Read the model definition and answer for the solid it produces. Units are mm, in the model's axes. A direction names the side the tool comes from. Give positions to 0.01 mm unless a question says otherwise; leave off trailing zeros. Order: outer loops, then holes, each group sorted by start corner. A loop starts at its lowest first (then second) coordinate and runs counter-clockwise, first axis right, second up. Notation, with made-up numbers: (83, -7) - (114, -7) arc R22 ccw to (114, 14) - close; hole circle Ø10 at (47, -6.75). An arc over 180 degrees is marked (long way). Return JSON: item names as keys, results as strings.
```python
from build123d import *

# Parameters (mm, degrees)
F0_R           = 20.05
F1_DEPTH       = 3.1
F2_R           = 10.05
F3_DEPTH       = 2
F4_R           = 0.5
F6_R           = 6
F7_DEPTH       = 10
F8_R           = 4.05
F9_DEPTH       = 8
F10_DEPTH      = 10.001
F10_DEPTH_BACK = 3.1010001
F11_T1_DEPTH   = 15.3170452501
F11_T4_ANGLE   = 359.9586190749


# Not quite as in the source:
# - a fillet or chamfer that OpenCascade refuses, or shapes differently, is made with other operations: its cross-section is extruded or revolved along the edge and cut away or added


with BuildPart() as f1:
    # F0 (on Top) → F1 (new body)
    with BuildSketch(Plane.XY):
        Circle(F0_R)
    extrude(amount=F1_DEPTH)

    # F2 (on face) → F3 (cut)
    with BuildSketch(Plane.XY.offset(3.1)):
        Circle(F2_R)
    extrude(amount=-F3_DEPTH, mode=Mode.SUBTRACT)

    # F4
    f4_edges = [f1.edges().sort_by_distance(p)[0] for p in [
        (-20.05, 0, 3.1),
        (-10.05, 0, 3.1),
        (-20.05, 0, 0),
    ]]
    fillet(f4_edges, radius=F4_R)

    # F6 (on face) → F7 (join)
    with BuildSketch(Plane(origin=(0, 0, 0), x_dir=(1, 0, 0), z_dir=(0, 0, -1))):
        Circle(F6_R)
    extrude(amount=F7_DEPTH)

    # F8 (on face) → F9 (cut)
    with BuildSketch(Plane(origin=(0, 0, -10), x_dir=(1, 0, 0), z_dir=(0, 0, -1))):
        Circle(F8_R)
    extrude(amount=-F9_DEPTH, mode=Mode.SUBTRACT)

    # F5 (on face) → F10 (cut, two sides)
    with BuildSketch(Plane(origin=(0, 0, 0), x_dir=(1, 0, 0), z_dir=(0, 0, -1))) as f10_sk:
        with BuildLine():
            Line((-2.5, 5), (-2.5, 0))
            ThreePointArc((-2.5, 0), (0, -2.5), (2.5, 0))
            Line((2.5, 0), (2.5, 5))
            ThreePointArc((2.5, 5), (1.9142135624, 6.4142135624), (0.5, 7))
            Line((0.5, 7), (-0.5, 7))
            ThreePointArc((-0.5, 7), (-1.9142135624, 6.4142135624), (-2.5, 5))
        make_face()
    extrude(amount=F10_DEPTH, mode=Mode.SUBTRACT)
    extrude(f10_sk.sketch, amount=-F10_DEPTH_BACK, mode=Mode.SUBTRACT)

    # F11: fillet of radius 1 on 3 edges, made by hand

    # F11_s2 → F11_t1 (cut)
    with BuildSketch(Plane.XY.offset(-15.3170452501)):
        with BuildLine():
            ThreePointArc((-4.2, -4.2848570571), (-3.1127016654, -4.49266866), (-2.5, -3.5707142143))
            Line((-2.5, -3.5707142143), (-2.4, -3.5707142143))
            ThreePointArc((-2.4, -3.5707142143), (-2.4, -5), (-2.3442646941, -5.4568235306))
            Line((-2.3442646941, -5.4568235306), (-2.4820201112, -5.5722146555))
            ThreePointArc((-2.4820201112, -5.5722146555), (-3.4303168121, -5.0440981918), (-4.27, -4.3562713414))
            Line((-4.27, -4.3562713414), (-4.2, -4.2848570571))
        make_face()
        with BuildLine():
            ThreePointArc((4.2, -4.2848570571), (3.1127016654, -4.49266866), (2.5, -3.5707142143))
            Line((2.5, -3.5707142143), (2.4, -3.5707142143))
            ThreePointArc((2.4, -3.5707142143), (2.4, -5), (2.3442646941, -5.4568235306))
            Line((2.3442646941, -5.4568235306), (2.4820201112, -5.5722146555))
            ThreePointArc((2.4820201112, -5.5722146555), (3.4303168121, -5.0440981918), (4.27, -4.3562713414))
            Line((4.27, -4.3562713414), (4.2, -4.2848570571))
        make_face()
    extrude(amount=F11_T1_DEPTH, mode=Mode.SUBTRACT)

    # F11_s3 → F11_t4 (revolve, cut)
    with BuildSketch(Plane(origin=(0, 0, 0), x_dir=(0, 0, 1), z_dir=(-0.9999999348, -0.0003611167, 0))):
        with BuildLine():
            ThreePointArc((-10, -5), (-9.7071067812, -5.7071067812), (-9, -6))
            Line((-9, -6), (-10, -6))
            Line((-10, -6), (-10, -5))
        make_face()
    revolve(axis=Axis((0, 0, -10), (0, 0, 1)), revolution_arc=F11_T4_ANGLE, mode=Mode.SUBTRACT)


solid = f1.part
```
Q1. Given pin 1 (1.5 mm diameter, centred on y = -3, z = -2, fed in from +X); pin 2 (16 mm diameter, centred on x = 0, y = 0, fed in from +Z); pin 3 (1.5 mm diameter, centred on y = -3, z = -2, fed in from -X), each flat-ended and moving along its own axis, determine where each tip first touches the part or whether it passes through.
Values:
{"pin 1": "stops at x = 5.56", "pin 2": "stops at z = 1.1", "pin 3": "stops at x = -5.56"}
Q2. A cutting plane is placed at A-A (x = 0). Write down the section's boundary in (y, z), and give its area (3 significant figures).
Values:
{"outline": "(-20.05, 0.5) arc R0.5 ccw to (-19.55, 0) - (-7, 0) - (-7, 1.1) - (-10.05, 1.1) - (-10.05, 2.6) arc R0.5 ccw to (-10.55, 3.1) - (-19.55, 3.1) arc R0.5 ccw to (-20.05, 2.6) - close; (2.5, -2) - (4.05, -2) - (4.05, -10) - (5, -10) arc R1 ccw to (6, -9) - (6, 0) - (19.55, 0) arc R0.5 ccw to (20.05, 0.5) - (20.05, 2.6) arc R0.5 ccw to (19.55, 3.1) - (10.55, 3.1) arc R0.5 ccw to (10.05, 2.6) - (10.05, 1.1) - (2.5, 1.1) - close", "area": "95.7 mm²"}
Q3. For faces 5 (the flat face through (2.5, -2.3, -1.6)), 6 (the cylindrical face through (0, 6, -4)), 7 (the flat face through (8, -8, 3.1)), 8 (the cylindrical face through (-3.13, -4.5, -5.07)), 9 (the flat face through (2, 2, 1.1)), determine the directions among +Z, -Z, +X, -X, +Y, -Y from which every point of the face is accessible in a straight line to the end or side of a thin tool.
Values:
{"face 5": "+Z, -Z", "face 6": "-Z", "face 7": "+Z, +X, -X, +Y, -Y", "face 8": "-Z, -Y", "face 9": "+Z"}
Q4. A cutting plane is placed at B-B (z = -1). Write down the section's boundary in (x, y), and give its area (3 significant figures).
Values:
{"outline": "(-4.2, -4.28) arc R1 ccw to (-2.5, -3.57) - (-2.5, 0) arc R2.5 cw to (2.5, 0) - (2.5, -3.57) arc R1 ccw to (4.2, -4.28) arc R6 ccw (long way) to start", "area": "72.4 mm²"}
Q5. Consider L1, parallel to X at y = 0, z = -6; L2, parallel to Y at x = 0, z = 1.85; L3, parallel to Z at x = -7, y = 15. Determine where each line is inside the solid, lowest interval first.
Values:
{"L1": "x = -6 to -4.05, 4.05 to 6", "L2": "y = -20.05 to -10.05, 10.05 to 20.05", "L3": "z = 0 to 3.1"}
Q6. A cutting plane is placed at C-C (z = -6). Write down the section's boundary in (x, y).
Values:
{"outline": "(-4.2, -4.28) arc R1 ccw to (-2.5, -3.57) - (-2.5, -3.19) arc R4.05 cw (long way) to (2.5, -3.19) - (2.5, -3.57) arc R1 ccw to (4.2, -4.28) arc R6 ccw (long way) to start"}
Q7. Determine the mould class of faces 1 (the cylindrical face through (-15.91, -12.2, 1.54)), 2 (the cylindrical face through (3.13, -4.5, -5.07)), 3 (the cylindrical face through (1.93, -6.4, 0.54)), 4 (the flat face through (-5, -4, 0)) for opening direction Y: released by +Y, released by -Y, zero draft, split by the parting line, or undercut.
Values:
{"face 1": "split by the parting line", "face 2": "released by -Y", "face 3": "undercut", "face 4": "zero draft"}
